Part model, mm, in its own coordinate system. Face numbers are marked on the shaded views. A direction names the side the tool comes from. Round coordinates to 2 decimals unless told otherwise and drop trailing zeros. Loops run counter-clockwise (first coordinate to the right, second up) from the corner with the lowest first, then second, coordinate; pieces in that order, holes last. Notation, with made-up numbers: M 48,28.5 L 86,28.5 A13 cw 86,48.5 Z; hole C -16,74.5 d11. An arc over 180 degrees is marked long. Answer as CSV lines item,"result". Start each with the question number.
Item 1: Band-saw the part on C-C (x = 27.5). Give the cut face in (y, z).
Item 2: Drop flat-ended pins along their axis: pin 1 Ø4 at (y, z) = (-5, -18) entering from -X; pin 2 Ø6 at (y, z) = (-5.5, 10) entering from +X; pin 3 Ø8 at (x, y) = (7, -17.5) entering from +Z. Give the stop position or say it passes through.
Item 3: Band-saw the part on B-B (z = -2). Count the separate pieces of the cut face and the enclosed holes in it, and give its area (3 significant figures).
Item 4: Mould opens along X. For the marked faces 1, 2 and 3 say: pulls with the +X half, pulls with the -X half, needs draft (parallel to the pull), parting line crosses it, or undercut.
Item 5: Which spindle directions (+Z, -Z, +X, -X, +Y, -Y) get a long thin tool onto all of the face, cutting with end or side? Do the marked faces 4 and 5. Say none if no direction does.
Item 6: Band-saw the part on A-A (y = 14). Give the cut face in (x, z).
Item 7: Wall check: line 1 (X direction, y = -19.5, z = -3); line 2 (X direction, y = -9, z = 1.5); line 3 (Y direction, x = 41, z = 8.5). Give the ranges that are in metal, low to high.
```python
from build123d import *

# Parameters (mm, degrees)
F0_R     = 10.347631
F0_R_2   = 8.717715
F1_DEPTH = 25
F2_DEPTH = 25
F3_SIZE  = 3
F4_R     = 2
F5_DEPTH = 5
F6_R     = 1
F7_SIZE  = 2


with BuildPart() as f1:
    # F0 (on Front) → F1 (new body)
    with BuildSketch(Plane.XZ):
        with BuildLine():
            ThreePointArc((4.109595, -24.251677), (18.789865, -15.873677), (24.597411, 0))
            ThreePointArc((24.597411, 0), (18.789865, 15.873677), (4.109595, 24.251677))
            ThreePointArc((4.109595, 24.251677), (-24.597411, 0), (4.109595, -24.251677))
        make_face()
        Circle(F0_R, mode=Mode.SUBTRACT)
        with BuildLine():
            ThreePointArc((4.109595, 24.251677), (18.789865, 15.873677), (24.597411, 0))
            ThreePointArc((24.597411, 0), (18.789865, -15.873677), (4.109595, -24.251677))
            Line((4.109595, -24.251677), (55.238279, -15.58761))
            ThreePointArc((55.238279, -15.58761), (36.787036, 0), (55.238279, 15.58761))
            Line((55.238279, 15.58761), (4.109595, 24.251677))
        make_face()
        with BuildLine():
            ThreePointArc((68.406691, 0), (64.673928, 10.202704), (55.238279, 15.58761))
            ThreePointArc((55.238279, 15.58761), (36.787036, 0), (55.238279, -15.58761))
            ThreePointArc((55.238279, -15.58761), (64.673928, -10.202704), (68.406691, 0))
        make_face()
        with Locations((52.596863, 0)):
            Circle(F0_R_2, mode=Mode.SUBTRACT)
    extrude(amount=F1_DEPTH)

    # F0 (on Front) → F2 (join)
    with BuildSketch(Plane.XZ):
        with BuildLine():
            ThreePointArc((4.109595, -24.251677), (18.789865, -15.873677), (24.597411, 0))
            ThreePointArc((24.597411, 0), (18.789865, 15.873677), (4.109595, 24.251677))
            ThreePointArc((4.109595, 24.251677), (-24.597411, 0), (4.109595, -24.251677))
        make_face()
        Circle(F0_R, mode=Mode.SUBTRACT)
    extrude(amount=-F2_DEPTH)

    # F3
    f3_edges = [f1.edges().sort_by_distance(p)[0] for p in [
        (-10.347631, 25, 0),
        (43.879148, 0, 0),
    ]]
    chamfer(f3_edges, length=F3_SIZE)

    # F4
    f4_edges = [f1.edges().sort_by_distance(p)[0] for p in [
        (-4.109595, 25, 24.251677),
    ]]
    fillet(f4_edges, radius=F4_R)

    # F0 (on Front) → F5 (join)
    with BuildSketch(Plane.XZ):
        with BuildLine():
            ThreePointArc((68.406691, 0), (64.673928, 10.202704), (55.238279, 15.58761))
            ThreePointArc((55.238279, 15.58761), (36.787036, 0), (55.238279, -15.58761))
            ThreePointArc((55.238279, -15.58761), (64.673928, -10.202704), (68.406691, 0))
        make_face()
        with Locations((52.596863, 0)):
            Circle(F0_R_2, mode=Mode.SUBTRACT)
    extrude(amount=-F5_DEPTH)

    # F6
    f6_edges = [f1.edges().sort_by_distance(p)[0] for p in [
        (49.955448, 5, 15.58761),
    ]]
    fillet(f6_edges, radius=F6_R)

    # F7
    f7_edges = [f1.edges().sort_by_distance(p)[0] for p in [
        (43.879148, 5, 0),
    ]]
    chamfer(f7_edges, length=F7_SIZE)


solid = f1.part
```
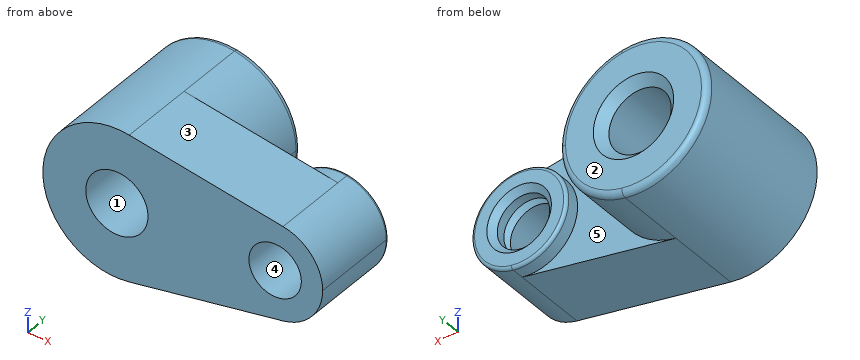
Answer block:
1,outline,"M -25,-20.29 L 0,-20.29 L 0,20.29 L -25,20.29 Z"
2,pin 1,"stops at x = -18.68"
2,pin 2,"stops at x = 66.77"
2,pin 3,"stops at z = 24.41"
3,separate pieces,"3"
3,enclosed holes,"0"
3,area,"2,150 mm^2"
4,face 1,"undercut"
4,face 2,"needs draft"
4,face 3,"pulls with the +X half"
5,face 4,"+Y, -Y"
5,face 5,"+Y"
6,outline,"M 4.11,-24.25 A24.6 ccw 24.6,0 A24.6 ccw 4.11,24.25 A24.6 ccw long Z; hole C 0,0 d20.7"
7,line 1,"x = -24.41 to -9.9, 9.9 to 44.41, 60.78 to 68.12"
7,line 2,"x = -24.55 to -10.24, 10.24 to 44.01, 61.18 to 68.34"
7,line 3,"y = -25 to 5"
